from build123d import *

# Parameters (mm, degrees)
EXTRUDE1_DEPTH = 193.675


with BuildPart() as part:
    # Sketch1 → Extrude1 (new body)
    with BuildSketch(Plane(origin=(0, 0, 0), x_dir=(1, 0, 0), z_dir=(0, 1, 0))):
        with BuildLine():
            Line((-198.4375, 65.0875), (-195.2625, 65.0875))
            ThreePointArc((-195.2625, 65.0875), (-186.282243879, 61.367756121), (-182.5625, 52.3875))
            Line((-182.5625, 52.3875), (-182.5625, -52.3875))
            ThreePointArc((-182.5625, -52.3875), (-186.282243879, -61.367756121), (-195.2625, -65.0875))
            Line((-195.2625, -65.0875), (-198.4375, -65.0875))
            Line((-198.4375, -65.0875), (-198.4375, -96.8375))
            Line((-198.4375, -96.8375), (198.4375, -96.8375))
            Line((198.4375, -96.8375), (198.4375, -65.0875))
            Line((198.4375, -65.0875), (195.2625, -65.0875))
            ThreePointArc((195.2625, -65.0875), (186.282243879, -61.367756121), (182.5625, -52.3875))
            Line((182.5625, -52.3875), (182.5625, 52.3875))
            ThreePointArc((182.5625, 52.3875), (186.282243879, 61.367756121), (195.2625, 65.0875))
            Line((195.2625, 65.0875), (198.4375, 65.0875))
            Line((198.4375, 65.0875), (198.4375, 96.8375))
            Line((198.4375, 96.8375), (-198.4375, 96.8375))
            Line((-198.4375, 96.8375), (-198.4375, 65.0875))
        make_face()
        with BuildLine():
            Line((-28.575, -65.0875), (-138.1125, -65.0875))
            ThreePointArc((-138.1125, -65.0875), (-147.092756121, -61.367756121), (-150.8125, -52.3875))
            Line((-150.8125, -52.3875), (-150.8125, 52.3875))
            ThreePointArc((-150.8125, 52.3875), (-147.092756121, 61.367756121), (-138.1125, 65.0875))
            Line((-138.1125, 65.0875), (-28.575, 65.0875))
            ThreePointArc((-28.575, 65.0875), (-19.594743879, 61.367756121), (-15.875, 52.3875))
            Line((-15.875, 52.3875), (-15.875, -52.3875))
            ThreePointArc((-15.875, -52.3875), (-19.594743879, -61.367756121), (-28.575, -65.0875))
        make_face(mode=Mode.SUBTRACT)
        with BuildLine():
            Line((138.1125, -65.0875), (28.575, -65.0875))
            ThreePointArc((28.575, -65.0875), (19.594743879, -61.367756121), (15.875, -52.3875))
            Line((15.875, -52.3875), (15.875, 52.3875))
            ThreePointArc((15.875, 52.3875), (19.594743879, 61.367756121), (28.575, 65.0875))
            Line((28.575, 65.0875), (138.1125, 65.0875))
            ThreePointArc((138.1125, 65.0875), (147.092756121, 61.367756121), (150.8125, 52.3875))
            Line((150.8125, 52.3875), (150.8125, -52.3875))
            ThreePointArc((150.8125, -52.3875), (147.092756121, -61.367756121), (138.1125, -65.0875))
        make_face(mode=Mode.SUBTRACT)
    extrude(amount=EXTRUDE1_DEPTH)


solid = part.part
Work out the finished part from the listing and answer in its coordinate system (mm). A direction names the side the tool comes from. Round coordinates to 2 decimals unless told otherwise and drop trailing zeros. Write each loop counter-clockwise with the first axis right and the second up, starting at its lowest first coordinate (ties: lowest second). Pieces come first, ordered by that corner, then holes. Notation, with made-up numbers: M 55,19 L 79,19 A28 cw 79,39 Z; hole C 2.5,52.25 d10. An arc over 180 degrees is marked long. Use a Markdown table: item, result.
1) The part is cut by section A-A on z = 16. Give the vertices of the cut face in (x, y) (1 decimal).
Taken from the geometry:
| item | result |
|---|---|
| outline | M -182.6,0 L -150.8,0 L -150.8,193.7 L -182.6,193.7 Z; M -15.9,0 L 15.9,0 L 15.9,193.7 L -15.9,193.7 Z; M 150.8,0 L 182.6,0 L 182.6,193.7 L 150.8,193.7 Z |
2) Flat-ended cylindrical pins translate along their axes: pin 1 (4 mm diameter, centred on y = 88, z = -12, fed in from +X); pin 2 (4 mm diameter, centred on y = 36.5, z = 7.5, fed in from -X); pin 3 (12 mm diameter, centred on y = 166, z = -54, fed in from -X). Find the tip coordinate at first contact, or state that the pin passes through.
Taken from the geometry:
| item | result |
|---|---|
| pin 1 | stops at x = 182.56 |
| pin 2 | stops at x = -182.56 |
| pin 3 | stops at x = -185.1 |
3) Consider line 1 (X direction, y = 123, z = -40.5) (1 decimal); line 2 (Z direction, x = -113, y = 123.5); line 3 (X direction, y = 105, z = -56.5). Determine where each line is inside the solid, lowest interval first. Write a range as [from, to].
Taken from the geometry:
| item | result |
|---|---|
| line 1 | x = [-182.6, -150.8], [-15.9, 15.9], [150.8, 182.6] |
| line 2 | z = [-96.84, -65.09], [65.09, 96.84] |
| line 3 | x = [-183.25, -150.13], [-16.56, 16.56], [150.13, 183.25] |
4) Which of the six approach directions +Z, -Z, +X, -X, +Y, -Y give full straight-line access (tool end or side, diameter ignored) to faces 5 (the face through (-186.184, 95.482, 61.268)), 6 (the face through (-3, 0, -1)), 7 (the face through (-147.19, 95.48, -61.27)), 8 (the face through (198.438, 95, -81)), 9 (the face through (186.382, 95.482, 61.466))?
Taken from the geometry:
| item | result |
|---|---|
| face 5 | -X, +Y, -Y |
| face 6 | +Z, -Z, +X, -X, -Y |
| face 7 | +Y, -Y |
| face 8 | +Z, -Z, +X, +Y, -Y |
| face 9 | +X, +Y, -Y |
5) Determine the mould class of faces 1 (the face through (-146.99, 95.48, 61.47)), 2 (the face through (15.875, 95, 1)), 3 (the face through (-3, 193.675, -1)), 4 (the face through (-198.438, 95, -81)) for opening direction X: pulls with the +X half, pulls with the -X half, needs draft (parallel to the pull), parting line crosses it, or undercut.
Taken from the geometry:
| item | result |
|---|---|
| face 1 | undercut |
| face 2 | undercut |
| face 3 | needs draft |
| face 4 | pulls with the -X half |
6) The part is cut by section D-D on z = -57. Give the vertices of the cut face in (x, y) (3 decimals), plus the area to 3 significant figures.
Taken from the geometry:
| item | result |
|---|---|
| outline | M -183.43,0 L -149.945,0 L -149.945,193.675 L -183.43,193.675 Z; M -16.742,0 L 16.742,0 L 16.742,193.675 L -16.742,193.675 Z; M 149.945,0 L 183.43,0 L 183.43,193.675 L 149.945,193.675 Z |
| area | 19,500 mm2 |
7) The part is cut by section C-C on x = 131. Give the vertices of the cut face in (y, z) (1 decimal).
Taken from the geometry:
| item | result |
|---|---|
| outline | M 0,-96.8 L 193.7,-96.8 L 193.7,-65.1 L 0,-65.1 Z; M 0,65.1 L 193.7,65.1 L 193.7,96.8 L 0,96.8 Z |
8) The part is cut by section B-B on y = 43.5. State how many separate pieces and enclosed holes the cut face has, plus the area to 3 significant figures.
Taken from the geometry:
| item | result |
|---|---|
| separate pieces | 1 |
| enclosed holes | 2 |
| area | 38,000 mm2 |
